Geometry: final body of the model. Coordinates: model frame, mm. A direction names the side the tool comes from. Coordinates: 2 decimals unless noted, no trailing zeros. Loops run counter-clockwise (first coordinate to the right, second up) from the corner with the lowest first, then second, coordinate; pieces in that order, holes last. Notation, with made-up numbers: M -13,1.5 L 23,1.5 A20 ccw 23,17.5 Z; hole C 5,21.25 d8. An arc over 180 degrees is marked long. Write each question's results on one line, items separated by ' | '. Start each with the question number.
from build123d import *

# Parameters (mm, degrees)
IZIM1_W                     = 90
IZIM1_H                     = 55
IZIM1_R                     = 1.65
Y_KSEKLIK_EKSTR_ZYON1_DEPTH = 1.55
IZIM2_W                     = 68.6
IZIM2_H                     = 4.5
Y_KSEKLIK_EKSTR_ZYON2_DEPTH = 17.8


with BuildPart() as part:
    # Çizim1 → Yükseklik-Ekstrüzyon1 (new body)
    with BuildSketch(Plane.XY):
        with Locations((45, -27.5)):
            Rectangle(IZIM1_W, IZIM1_H)
        with Locations(Location((86.15, -3.85, 0), (0, 0, 180))):
            Circle(IZIM1_R, mode=Mode.SUBTRACT)
        with Locations(Location((3.85, -51.15, 0), (0, 0, 180))):
            Circle(IZIM1_R, mode=Mode.SUBTRACT)
    extrude(amount=Y_KSEKLIK_EKSTR_ZYON1_DEPTH)

    # Çizim2 → Yükseklik-Ekstrüzyon2 (add)
    with BuildSketch(Plane.XY.offset(1.55)):
        with Locations((46, -2.25)):
            Rectangle(IZIM2_W, IZIM2_H)
    extrude(amount=Y_KSEKLIK_EKSTR_ZYON2_DEPTH)


solid = part.part
Item 1: Set-up query: faces 5 (the flat face through (80.3, -2, 10)), 6 (the flat face through (44, -27, 0)), 7 (the flat face through (46, -4.5, 10)). Return all of +Z, -Z, +X, -X, +Y, -Y with unobstructed straight access to the full face (end or side cutting, diameter ignored); none if empty.
Item 2: Section D-D, the plane y = -44. Return loops of the section in (x, z), plus the area to 4 significant figures.
Item 3: Ray query, L1, parallel to Y at x = 3.85, z = 0.9; L2, parallel to X at y = -51.15, z = 0.7; L3, parallel to X at y = -3.85, z = 0.75. Return the intervals inside material, ascending. Write a range as [from, to].
Item 4: Section C-C, the plane z = 16.75. Return loops of the section in (x, y).
Item 5: Pull-direction query (X, two-part tool) for faces 1 (the flat face through (44, 0, 10)), 2 (the flat face through (11.7, -2, 10)), 3 (the cylindrical face through (3.089, -49.686, 0.764)), 4 (the cylindrical face through (84.576, -4.346, 0.764)); classes: released by +X, released by -X, zero draft, split by the parting line, or undercut.
Item 6: Section B-B, the plane x = 77.5. Return loops of the section in (y, z).
Item 7: Contact query for flat-ended pins moving along their axis: P1, Ø1.5, axis at x = 41, y = -7.5, coming from the +Z side; P2, Ø3.5, axis at y = -2.5, z = 12, coming from the +X side; P3, Ø2, axis at y = -3.5, z = 11, coming from the -X side. Output: stop coordinate, or through.
Item 8: Section A-A, the plane x = 3.85. Return loops of the section in (y, z), plus the area to 3 significant figures.
Solutions:
1) face 5: +Z, +X, +Y, -Y | face 6: -Z, +X, -X, +Y, -Y | face 7: +Z, +X, -X, -Y
2) outline: M 0,0 L 90,0 L 90,1.55 L 0,1.55 Z | area: 139.5 mm²
3) L1: y = [-55, -52.8], [-49.5, 0] | L2: x = [0, 2.2], [5.5, 90] | L3: x = [0, 84.5], [87.8, 90]
4) outline: M 11.7,-4.5 L 80.3,-4.5 L 80.3,0 L 11.7,0 Z
5) face 1: zero draft | face 2: released by -X | face 3: undercut | face 4: undercut
6) outline: M -55,0 L 0,0 L 0,19.35 L -4.5,19.35 L -4.5,1.55 L -55,1.55 Z
7) P1: stops at z = 1.55 | P2: stops at x = 80.3 | P3: stops at x = 11.7
8) outline: M -55,0 L -52.8,0 L -52.8,1.55 L -55,1.55 Z; M -49.5,0 L 0,0 L 0,1.55 L -49.5,1.55 Z | area: 80.1 mm²
